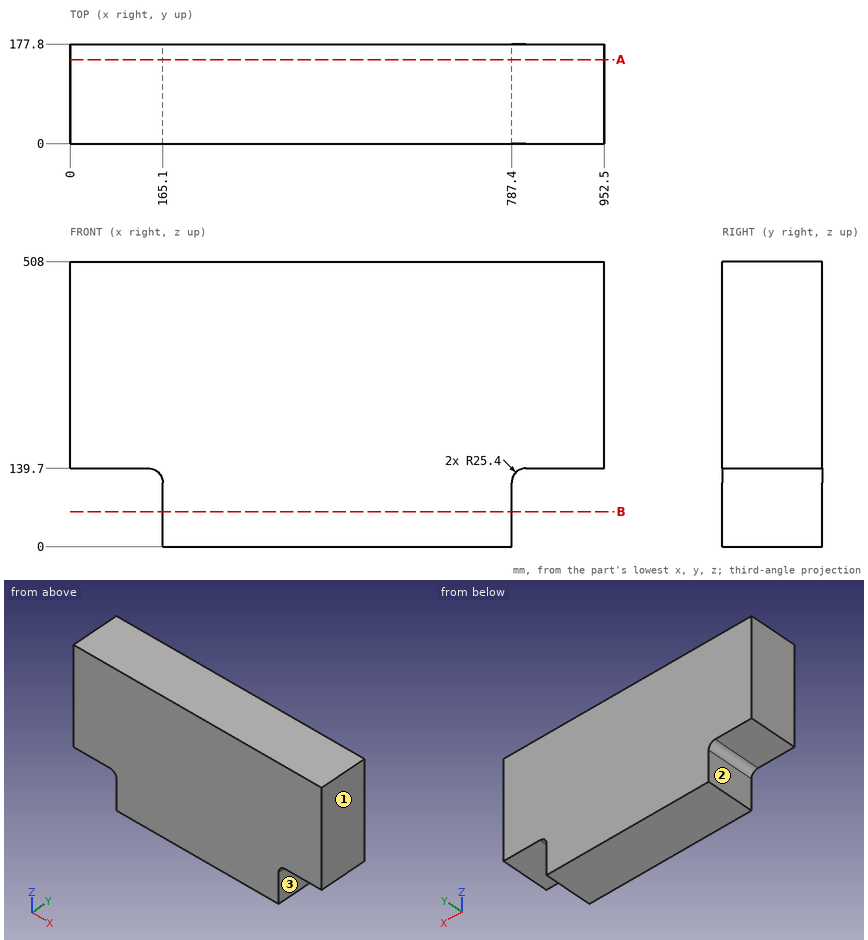
Study the drawing (mm; zero at the part's minimum x, y, z) and answer. A direction names the side the tool comes from. Coordinates: 2 decimals unless noted, no trailing zeros. Write each loop counter-clockwise with the first axis right and the second up, starting at its lowest first coordinate (ties: lowest second). Pieces come first, ordered by that corner, then holes. Notation, with made-up numbers: M 47.5,21 L 69.5,21 A9 cw 69.5,34 Z; hole C 7.25,35 d9. An arc over 180 degrees is marked long. Use a Markdown table: item, result. Add a question column.
1. Which of the six approach directions +Z, -Z, +X, -X, +Y, -Y give full straight-line access (tool end or side, diameter ignored) to the marked faces 1, 2 and 3?
2. Straight lines are drawn through the part: line 1 along Z through (x, y) = (894, 81); line 2 along X through (y, z) = (22.5, 34); line 3 along X through (y, z) = (62, 123.5). For each, find the intervals that lie inside material, in ascending order. Write a range as [from, to].
3. Section B-B (z = 62.5) is taken. Give the vertices of the cut face in (x, y).
4. Section A-A (y = 150) is taken. Give the vertices of the cut face in (x, z).
5. Given P1, Ø10, axis at x = 826.5, y = 159.5, coming from the -Z side, flat-ended and moving along its own axis, determine where the tip first touches the part or whether it passes through.
Data:
| question | item | result |
|---|---|---|
| 1 | face 1 | +Z, -Z, +X, +Y, -Y |
| 1 | face 2 | -Z, -X, +Y, -Y |
| 1 | face 3 | -Z, +X, +Y, -Y |
| 2 | line 1 | z = [139.7, 508] |
| 2 | line 2 | x = [165.1, 787.4] |
| 2 | line 3 | x = [163.38, 789.12] |
| 3 | outline | M 165.1,0 L 787.4,0 L 787.4,177.8 L 165.1,177.8 Z |
| 4 | outline | M 0,139.7 L 139.7,139.7 A25.4 cw 165.1,114.3 L 165.1,0 L 787.4,0 L 787.4,114.3 A25.4 cw 812.8,139.7 L 952.5,139.7 L 952.5,508 L 0,508 Z |
| 5 | P1 | stops at z = 139.7 |
